Build history of the part. All positions in model axes, mm. A direction names the side the tool comes from. Coordinates: 2 decimals unless noted, no trailing zeros. Loops run counter-clockwise (first coordinate to the right, second up) from the corner with the lowest first, then second, coordinate; pieces in that order, holes last. Notation, with made-up numbers: M 73,-5 L 80,-5 A23 cw 80,4 Z; hole C 18,52 d2. An arc over 180 degrees is marked long. Write each question's results on one line, items separated by ' | '. Start each with the question number.
from build123d import *

# Parameters (mm, degrees)
EXTRUSION4_DEPTH        = 7.5
ESQUISSE2_R             = 3.25
ENL_V_MAT_EXTRU_1_DEPTH = 15


with BuildPart() as part:
    # Esquisse1 → Extrusion4 (new, symmetric)
    with BuildSketch(Plane.XY):
        with BuildLine():
            Line((-30.026499529, -11.063874821), (-11.335566656, -61.789619296))
            ThreePointArc((-11.335566656, -61.789619296), (-10.845370144, -62.539560252), (-10.076944424, -63.000240152))
            Line((-10.076944424, -63.000240152), (-7.301265108, -63.902113033))
            ThreePointArc((-7.301265108, -63.902113033), (-6.996100049, -63.975376681), (-6.683231119, -64))
            Line((-6.683231119, -64), (7, -64))
            Line((7, -64), (7, -65.4))
            Line((7, -65.4), (-6.683231119, -65.4))
            ThreePointArc((-6.683231119, -65.4), (-7.2151083, -65.358140358), (-7.7338889, -65.233592155))
            Line((-7.7338889, -65.233592155), (-10.509568216, -64.331719275))
            ThreePointArc((-10.509568216, -64.331719275), (-11.81589194, -63.548563445), (-12.64922601, -62.27366382))
            Line((-12.64922601, -62.27366382), (-31.340158883, -11.547919345))
            ThreePointArc((-31.340158883, -11.547919345), (0.161979155, 33.399607225), (31.226678681, -11.851351759))
            Line((31.226678681, -11.851351759), (12.649044499, -60.800857693))
            ThreePointArc((12.649044499, -60.800857693), (11.815350768, -62.056270768), (10.520938582, -62.828024819))
            Line((10.520938582, -62.828024819), (7.7338889, -63.733592155))
            ThreePointArc((7.7338889, -63.733592155), (7.2151083, -63.858140358), (6.683231119, -63.9))
            Line((6.683231119, -63.9), (-7, -63.9))
            Line((-7, -63.9), (-7, -62.5))
            Line((-7, -62.5), (6.683231119, -62.5))
            ThreePointArc((6.683231119, -62.5), (6.996100049, -62.475376681), (7.301265108, -62.402113033))
            Line((7.301265108, -62.402113033), (10.08831479, -61.496545697))
            ThreePointArc((10.08831479, -61.496545697), (10.849733723, -61.042572725), (11.3401418, -60.304094446))
            Line((11.3401418, -60.304094446), (29.917775982, -11.354588512))
            ThreePointArc((29.917775982, -11.354588512), (0.155189609, 31.999623688), (-30.026499529, -11.063874821))
        make_face()
    extrude(amount=EXTRUSION4_DEPTH, both=True)

    # Esquisse2 → Enl_v. mat.-Extru.1 (cut)
    with BuildSketch(Plane.XZ.offset(65.4)):
        with Locations(Location((0, 0, 0), (0, 0, 270))):
            Circle(ESQUISSE2_R)
    extrude(amount=-ENL_V_MAT_EXTRU_1_DEPTH, mode=Mode.SUBTRACT)


solid = part.part
1. Wall check: line 1 along Y through (x, z) = (7.5, 3.75); line 2 along X through (y, z) = (-32.5, -1.25); line 3 along X through (y, z) = (8.5, 0.5). Give the ranges that are in metal, low to high.
2. Band-saw the part on A-A, the plane x = 0. List the corners of the cut face in (y, z), plus the area to 3 significant figures.
3. Which spindle directions (+Z, -Z, +X, -X, +Y, -Y) get a long thin tool onto all of the face, cutting with end or side? Do faces 4 (the flat face through (-25, -27, 7.5)), 5 (the flat face through (-0.3, -62.5, 3.4)). Say none if no direction does.
4. Mould opens along Y. For faces 1 (the flat face through (-8.709, -63.445, 0.105)), 2 (the cylindrical face through (-1.978, -64.71, 2.579)), 3 (the flat face through (0.3, -65.4, 3.4)) say: +Y half, -Y half, draft (parallel to the pull), parting line (faces both ways), or undercut.
5. Band-saw the part on D-D, the plane x = -16. List the corners of the cut face in (y, z), plus the area to 3 significant figures.
6. Band-saw the part on C-C, the plane z = 0. Give the number of separate pieces and of enclosed holes in the cut face, plus the area to 3 significant figures.
7. Pin check, flat tips, straight feed: pin 1 (7 mm diameter, centred on x = -0.5, z = -1.5, fed in from -Y); pin 2 (5 mm diameter, centred on x = 0, z = 0, fed in from -Y); pin 3 (1 mm diameter, centred on y = 11, z = -2, fed in from -X); pin 4 (2 mm diameter, centred on y = 19, z = -4.5, fed in from +X). Stop position of each tip, or through.
8. Band-saw the part on B-B, the plane y = 0. List the corners of the cut face in (x, z).
Checked values:
1) line 1: -63.8 to -62.34, 31.11 to 32.55 | line 2: -23.62 to -22.13, 21.89 to 23.39 | line 3: -32.3 to -30.85, 30.85 to 32.3
2) outline: M -65.4,-7.5 L -64,-7.5 L -64,-3.25 L -65.4,-3.25 Z; M -65.4,3.25 L -64,3.25 L -64,7.5 L -65.4,7.5 Z; M -63.9,-7.5 L -62.5,-7.5 L -62.5,-3.25 L -63.9,-3.25 Z; M -63.9,3.25 L -62.5,3.25 L -62.5,7.5 L -63.9,7.5 Z; M 32,-7.5 L 33.4,-7.5 L 33.4,7.5 L 32,7.5 Z | area: 44.8 mm²
3) face 4: +Z, +X, -X, +Y, -Y | face 5: +Z, -Z
4) face 1: undercut | face 2: draft | face 3: -Y half
5) outline: M -53.18,-7.5 L -49.13,-7.5 L -49.13,7.5 L -53.18,7.5 Z; M 27.71,-7.5 L 29.32,-7.5 L 29.32,7.5 L 27.71,7.5 Z | area: 84.8 mm²
6) separate pieces: 3 | enclosed holes: 0 | area: 363 mm²
7) pin 1: y = -65.4 | pin 2: y = 31.9 | pin 3: x = -31.71 | pin 4: x = 28.13
8) outline: M -33.4,-7.5 L -32,-7.5 L -32,7.5 L -33.4,7.5 Z; M 32,-7.5 L 33.4,-7.5 L 33.4,7.5 L 32,7.5 Z
